For this review, take the finished solid that the model builds, in its own axes (mm). A direction names the side the tool comes from. Give positions to 0.01 mm unless a question says otherwise; leave off trailing zeros. Order: outer loops, then holes, each group sorted by start corner. A loop starts at its lowest first (then second) coordinate and runs counter-clockwise, first axis right, second up. Notation, with made-up numbers: (46, 43.5) - (101, 43.5) arc R23 cw to (101, 58.5) - close; hole circle Ø3 at (57, 3.5). An arc over 180 degrees is marked (long way). Use a Markdown table: item, result. Add a question column.
1) We need section A-A on x = 18. Write out the cut boundary in (y, z).
2) We need section C-C on y = 4.6. Write out the cut boundary in (x, z).
3) Mouldability with a two-part tool opening along Z and no side actions: class faces 1 (the face through (0, 0, -12)), 2 (the face through (-0.488, 2.859, 13.804)), 3 (the face through (0, 3, -20)) as released by +Z, released by -Z, zero draft, split by the parting line, or undercut.
4) We need section D-D on z = -2.5. Write out the cut boundary in (x, y).
5) Wall thickness on L1, parallel to Z at x = 0, y = 2.95; L2, parallel to Z at x = -24.5, y = 2.65; L3, parallel to X at y = 5, z = 2: over which ranges is each line inside the solid? List them lowest first.
6) Clearance check with flat-ended pins moving along their axes: P1, Ø1.7, axis at x = 15, y = 1.5, coming from the +Z side; P2, Ø3, axis at x = 25, z = 7, coming from the -Y side; P3, Ø1.7, axis at x = 22.5, y = 3.5, coming from the -Z side. State where each tip first meets the part, or that it passes through.
7) We need section B-B on x = 0. Write out the cut boundary in (y, z), then the cut area to 3 significant figures.
8) Machinability: for faces 4 (the face through (-20, 3, -16)), 5 (the face through (0, 3, 10.5)), 6 (the face through (20.5, 5, -7)), which of the approach directions +Z, -Z, +X, -X, +Y, -Y give a long, thin tool a straight path to every point of the face, cutting with its end or side? Answer none if there is none.
```python
from build123d import *

# Parameters (mm, degrees)
RESSALTO_EXTRUS_O1_DEPTH = 5.8
ESBO_O2_W                = 41
ESBO_O2_H                = 21
CORTE_EXTRUS_O1_DEPTH    = 37.519036132
FILETE1_R                = 6
ESBO_O4_W                = 57
ESBO_O4_H                = 21
CORTE_EXTRUS_O2_DEPTH    = 4
ESBO_O5_W                = 16
ESBO_O5_H                = 8.8
CORTE_EXTRUS_O3_DEPTH    = 10


with BuildPart() as part:
    # Esboço1 → Ressalto-extrusão1 (new body)
    with BuildSketch(Plane(origin=(0, 0, 0), x_dir=(1, 0, 0), z_dir=(0, 1, 0))):
        with BuildLine():
            Line((-4, 20), (-4, 16))
            Line((-4, 16), (-2.25, 16))
            ThreePointArc((-2.25, 16), (0, 18.25), (2.25, 16))
            Line((2.25, 16), (4, 16))
            Line((4, 16), (4, 20))
            Line((4, 20), (-4, 20))
        make_face()
        with BuildLine():
            Line((-2.25, 16), (-4, 16))
            Line((-4, 16), (-4, 12))
            Line((-4, 12), (4, 12))
            Line((4, 12), (4, 16))
            Line((4, 16), (2.25, 16))
            ThreePointArc((2.25, 16), (0, 13.75), (-2.25, 16))
        make_face()
        Polygon((-30, 16), (-30, -16), (-4, -16), (-4, -12), (4, -12), (4, -16), (30, -16), (30, 16), (4, 16), (4, 12), (-4, 12), (-4, 16), align=None)
        with BuildLine():
            Line((-4, -12), (-4, -16))
            Line((-4, -16), (-2.25, -16))
            ThreePointArc((-2.25, -16), (0, -13.75), (2.25, -16))
            Line((2.25, -16), (4, -16))
            Line((4, -16), (4, -12))
            Line((4, -12), (-4, -12))
        make_face()
        with BuildLine():
            Line((-2.25, -16), (-4, -16))
            Line((-4, -16), (-4, -20))
            Line((-4, -20), (4, -20))
            Line((4, -20), (4, -16))
            Line((4, -16), (2.25, -16))
            ThreePointArc((2.25, -16), (0, -18.25), (-2.25, -16))
        make_face()
    extrude(amount=RESSALTO_EXTRUS_O1_DEPTH)

    # Esboço2 → Corte-extrusão1 (cut, through all)
    with BuildSketch(Plane(origin=(0, 5.8, 0), x_dir=(1, 0, 0), z_dir=(0, 1, 0))):
        Rectangle(ESBO_O2_W, ESBO_O2_H)
    extrude(amount=-CORTE_EXTRUS_O1_DEPTH, mode=Mode.SUBTRACT)

    # Filete1
    # the kernel refuses this fillet: 6 mm, written as the material it adds along each edge
    with BuildSketch(Plane(origin=(4, 0, -16), x_dir=(0, 0, -1), z_dir=(0, 1, 0))) as filete1_piece_1:
        with BuildLine():
            CenterArc((6, -5.656854249), FILETE1_R, 109.471220634, 70.528779366)
            Line((0, -5.656854249), (-0.12, -5.656854249))
            Line((-0.12, -5.656854249), (-0.12, 0))
            Line((-0.12, 0), (0, 0.12))
            ThreePointArc((0, 0.12), (2, 0.12), (3.96, 0.113137085))
            Line((3.96, 0.113137085), (4, 0))
        make_face()
    extrude(amount=5.8)
    with BuildSketch(Plane(origin=(-4, 0, -16), x_dir=(0, 0, -1), z_dir=(0, 1, 0))) as filete1_piece_2:
        with BuildLine():
            CenterArc((6, 5.656854249), FILETE1_R, 180, 70.528779366)
            Line((0, 5.656854249), (-0.12, 5.656854249))
            Line((-0.12, 5.656854249), (-0.12, 0))
            Line((-0.12, 0), (0, -0.12))
            ThreePointArc((0, -0.12), (2, -0.12), (3.96, -0.113137085))
            Line((3.96, -0.113137085), (4, 0))
        make_face()
    extrude(amount=5.8)
    with BuildSketch(Plane(origin=(-4, 0, 16), x_dir=(-1, 0, 0), z_dir=(0, 1, 0))) as filete1_piece_3:
        with BuildLine():
            CenterArc((5.656854249, 6), FILETE1_R, 199.471220634, 70.528779366)
            Line((0, 4), (-0.113137085, 3.96))
            ThreePointArc((-0.113137085, 3.96), (-0.12, 2), (-0.12, 0))
            Line((-0.12, 0), (0, -0.12))
            Line((0, -0.12), (5.656854249, -0.12))
            Line((5.656854249, -0.12), (5.656854249, 0))
        make_face()
    extrude(amount=5.8)
    with BuildSketch(Plane(origin=(4, 0, 16), x_dir=(1, 0, 0), z_dir=(0, 1, 0))) as filete1_piece_4:
        with BuildLine():
            CenterArc((5.656854249, -6), FILETE1_R, 90, 70.528779366)
            Line((0, -4), (-0.113137085, -3.96))
            ThreePointArc((-0.113137085, -3.96), (-0.12, -2), (-0.12, 0))
            Line((-0.12, 0), (0, 0.12))
            Line((0, 0.12), (5.656854249, 0.12))
            Line((5.656854249, 0.12), (5.656854249, 0))
        make_face()
    extrude(amount=5.8)

    # Esboço4 → Corte-extrusão2 (cut)
    with BuildSketch(Plane.XZ):
        Rectangle(ESBO_O4_W, ESBO_O4_H)
    extrude(amount=-CORTE_EXTRUS_O2_DEPTH, mode=Mode.SUBTRACT)

    # Esboço5 → Corte-extrusão3 (cut)
    with BuildSketch(Plane.XZ.offset(-4)):
        with Locations((20.5, 0)):
            Rectangle(ESBO_O5_W, ESBO_O5_H)
    extrude(amount=-CORTE_EXTRUS_O3_DEPTH, mode=Mode.SUBTRACT)


solid = part.part
```
Checked values:
| question | item | result |
|---|---|---|
| 1 | outline | (0, -16) - (5.8, -16) - (5.8, -10.5) - (0, -10.5) - close; (0, 10.5) - (5.8, 10.5) - (5.8, 16) - (0, 16) - close |
| 2 | outline | (-30, -16) - (-9.66, -16) arc R6 cw to (-4, -20) - (4, -20) arc R6 cw to (9.66, -16) - (30, -16) - (30, 16) - (9.66, 16) arc R6 cw to (4, 20) - (-4, 20) arc R6 cw to (-9.66, 16) - (-30, 16) - close; hole (-20.5, -10.5) - (20.5, -10.5) - (20.5, -4.4) - (28.5, -4.4) - (28.5, 4.4) - (20.5, 4.4) - (20.5, 10.5) - (-20.5, 10.5) - close; hole circle Ø4.5 at (0, -16); hole circle Ø4.5 at (0, 16) |
| 3 | face 1 | zero draft |
| 3 | face 2 | undercut |
| 3 | face 3 | released by -Z |
| 4 | outline | (-30, 0) - (-28.5, 0) - (-28.5, 4) - (-20.5, 4) - (-20.5, 5.8) - (-30, 5.8) - close; (28.5, 0) - (30, 0) - (30, 5.8) - (28.5, 5.8) - close |
| 5 | L1 | -20 to -18.25, -13.75 to -10.5, 10.5 to 13.75, 18.25 to 20 |
| 5 | L2 | -16 to -10.5, 10.5 to 16 |
| 5 | L3 | -30 to -20.5, 28.5 to 30 |
| 6 | P1 | z = 16 |
| 6 | P2 | y = 4 |
| 6 | P3 | z = -16 |
| 7 | outline | (0, -20) - (5.8, -20) - (5.8, -18.25) - (0, -18.25) - close; (0, -13.75) - (5.8, -13.75) - (5.8, -10.5) - (0, -10.5) - close; (0, 10.5) - (5.8, 10.5) - (5.8, 13.75) - (0, 13.75) - close; (0, 18.25) - (5.8, 18.25) - (5.8, 20) - (0, 20) - close |
| 7 | area | 58.0 mm² |
| 8 | face 4 | -Z, -X, +Y, -Y |
| 8 | face 5 | -Y |
| 8 | face 6 | +Y, -Y |
